Verification items for this drawing (mm, ordinates from the low corner). Round coordinates to 2 decimals unless told otherwise and drop trailing zeros. Loops run counter-clockwise (first coordinate to the right, second up) from the corner with the lowest first, then second, coordinate; pieces in that order, holes last. Notation, with made-up numbers: M -11,17.25 L 1,17.25 A32 cw 1,52.25 Z; hole C 80.5,33.5 d9. An arc over 180 degrees is marked long. Write item = value, one per line. Start each with the question number.
(1) Go/stop test with flat-tipped pins: P1, Ø6, axis at x = 13.5, z = 267, coming from the +Y side (1 decimal); P2, Ø1.5, axis at x = 33, z = 163.5, coming from the -Y side (1 decimal); P3, Ø4, axis at x = 30, y = 10.5, coming from the -Z side; P4, Ø1, axis at y = 28.5, z = 140, coming from the +X side. Record where each tip stops, or that it passes through.
(2) Cross-section at C-C on z = 73.5. Record the boundary of the cut face in (x, y) (1 decimal).
(3) Scan lines: L1, parallel to X at y = 19, z = 181.5; L2, parallel to Y at x = 29, z = 91.5. Record each from-to range of solid material in increasing order. Write a range as from..to.
(4) Cross-section at B-B on x = 28. Record the boundary of the cut face in (y, z), plus the area to 3 significant figures.
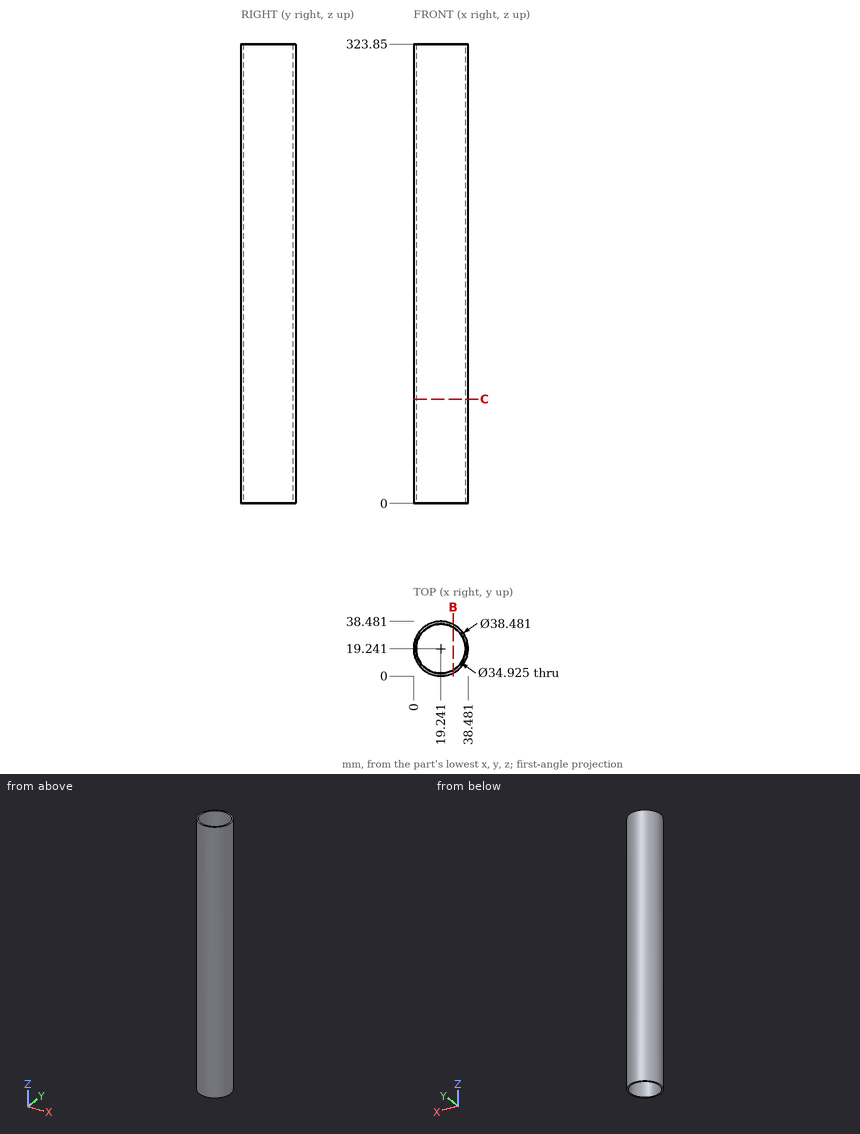
Result:
q1.P1 = 38.3
q1.P2 = 5.1
q1.P3 = through
q1.P4 = 36.37
q2.outline = C 19.2,19.2 d38.5; hole C 19.2,19.2 d34.9
q3.L1 = 0..1.78, 36.7..38.48
q3.L2 = 2.66..4.76, 33.72..35.82
q4.outline = M 2.11,0 L 4.13,0 L 4.13,323.85 L 2.11,323.85 Z; M 34.35,0 L 36.37,0 L 36.37,323.85 L 34.35,323.85 Z
q4.area = 1,310 mm^2
